Check sheet for the modelled part. Datum: model origin and axes. Units: mm. Face numbers are marked on the shaded views. A direction names the side the tool comes from. Round coordinates to 2 decimals unless told otherwise and drop trailing zeros. Write each loop counter-clockwise with the first axis right and the second up, starting at its lowest first coordinate (ties: lowest second). Pieces come first, ordered by that corner, then holes.
from build123d import *

# Parameters (mm, degrees)
BOSS_EXTRUDE1_DEPTH      = 12.5
BOSS_EXTRUDE1_DEPTH_BACK = 2.5
F_3DSKETCH2_R            = 4.5
CUT_EXTRUDE2_DEPTH       = 1
CUT_EXTRUDE3_REACH       = 68.802
SKETCH3_R                = 3.75
CUT_EXTRUDE6_OUTLINE_R   = 3.25
CUT_EXTRUDE6_DEPTH       = 10
CUT_EXTRUDE7_DEPTH       = 2.5
FILLET1_R                = 5
FILLET2_R                = 4
FILLET3_R                = 4
FILLET4_R                = 3
FILLET5_R                = 3
FILLET6_R                = 4


# Read off the part's stored shape, not the designer's step: Cut-Extrude6
with BuildPart() as part:
    # Sketch1 → Boss-Extrude1 (new, two sides: drawn at the far end of the back side and taken through both)
    with BuildSketch(Plane.XY.offset(-BOSS_EXTRUDE1_DEPTH_BACK)):
        Polygon((0, -8), (0, -32), (-3.5, -32), (-3.5, -64), (0, -64), (0, -38), (7, -38), (7, -20), (12, -20), (12, -8), align=None)
    extrude(amount=BOSS_EXTRUDE1_DEPTH + BOSS_EXTRUDE1_DEPTH_BACK)

    # 3DSketch2 → Cut-Extrude2 (cut)
    with BuildSketch(Plane(origin=(-3.5, -54, 5), x_dir=(0, -1, 0), z_dir=(-1, 0, 0))):
        with Locations(Location((0, 0, 0), (0, 0, 270))):
            Circle(F_3DSKETCH2_R)
    extrude(amount=-CUT_EXTRUDE2_DEPTH, mode=Mode.SUBTRACT)

    # Sketch3 → Cut-Extrude3 (cut, up to next)
    with BuildSketch(Plane.ZY.offset(2.5), mode=Mode.PRIVATE) as cut_extrude3_sk1:
        with Locations((5, -54)):
            Circle(SKETCH3_R)
    cut_extrude3_tool1 = extrude(cut_extrude3_sk1.sketch, amount=-CUT_EXTRUDE3_REACH, mode=Mode.PRIVATE) & part.part
    add(cut_extrude3_tool1.solids().sort_by_distance((-2.5, -54, 5))[0], mode=Mode.SUBTRACT)

    # Cut-Extrude6 outline → Cut-Extrude6 (cut)
    with BuildSketch(Plane.YZ):
        with Locations((-16.5, 5)):
            Circle(CUT_EXTRUDE6_OUTLINE_R)
    extrude(amount=CUT_EXTRUDE6_DEPTH, mode=Mode.SUBTRACT)

    # Sketch4 → Cut-Extrude7 (cut)
    with BuildSketch(Plane.ZY.offset(3.5)):
        with BuildLine():
            Line((5, -46.75), (5, -45.75))
            ThreePointArc((5, -45.75), (4.24685511, -45.784449332), (3.5, -45.88750963))
            Line((3.5, -45.88750963), (3.5, -46.75))
            Line((3.5, -46.75), (5, -46.75))
        make_face()
        with BuildLine():
            ThreePointArc((6.5, -45.88750963), (5.75314489, -45.784449332), (5, -45.75))
            Line((5, -45.75), (5, -46.75))
            Line((5, -46.75), (6.5, -46.75))
            Line((6.5, -46.75), (6.5, -45.88750963))
        make_face()
    extrude(amount=-CUT_EXTRUDE7_DEPTH, mode=Mode.SUBTRACT)

    # Fillet1
    # the kernel refuses this fillet: 5 mm, written as the material it takes off along each edge
    with BuildSketch(Plane(origin=(7, -38, -15), x_dir=(-1, 0, 0), z_dir=(0, 0, 1))) as fillet1_piece_1:
        with BuildLine():
            CenterArc((FILLET1_R, -FILLET1_R), FILLET1_R, 90, 90)
            Line((0, -FILLET1_R), (-FILLET1_R * 0.02, -FILLET1_R))
            Line((-FILLET1_R * 0.02, -FILLET1_R), (-FILLET1_R * 0.02, FILLET1_R * 0.02))
            Line((-FILLET1_R * 0.02, FILLET1_R * 0.02), (FILLET1_R, FILLET1_R * 0.02))
            Line((FILLET1_R, FILLET1_R * 0.02), (FILLET1_R, 0))
        make_face()
    extrude(amount=40, mode=Mode.SUBTRACT)
    with BuildSketch(Plane(origin=(24.5, -8, 12.5), x_dir=(0, 0, -1), z_dir=(-1, 0, 0))) as fillet1_piece_2:
        with BuildLine():
            CenterArc((FILLET1_R, FILLET1_R), FILLET1_R, 180, 90)
            Line((0, FILLET1_R), (-FILLET1_R * 0.02, FILLET1_R))
            Line((-FILLET1_R * 0.02, FILLET1_R), (-FILLET1_R * 0.02, -FILLET1_R * 0.02))
            Line((-FILLET1_R * 0.02, -FILLET1_R * 0.02), (FILLET1_R, -FILLET1_R * 0.02))
            Line((FILLET1_R, -FILLET1_R * 0.02), (FILLET1_R, 0))
        make_face()
    extrude(amount=37, mode=Mode.SUBTRACT)
    with BuildSketch(Plane(origin=(24.5, -8, -2.5), x_dir=(0, 0, 1), z_dir=(-1, 0, 0))) as fillet1_piece_3:
        with BuildLine():
            CenterArc((FILLET1_R, -FILLET1_R), FILLET1_R, 90, 90)
            Line((0, -FILLET1_R), (-FILLET1_R * 0.02, -FILLET1_R))
            Line((-FILLET1_R * 0.02, -FILLET1_R), (-FILLET1_R * 0.02, FILLET1_R * 0.02))
            Line((-FILLET1_R * 0.02, FILLET1_R * 0.02), (FILLET1_R, FILLET1_R * 0.02))
            Line((FILLET1_R, FILLET1_R * 0.02), (FILLET1_R, 0))
        make_face()
    extrude(amount=37, mode=Mode.SUBTRACT)
    with BuildSketch(Plane(origin=(-3.5, -32, -14.424240018), x_dir=(1, 0, 0), z_dir=(0, 0, 1))) as fillet1_piece_4:
        with BuildLine():
            CenterArc((5, -4.769696007), FILLET1_R, 107.457603124, 72.542396876)
            Line((0, -4.769696007), (-0.1, -4.769696007))
            Line((-0.1, -4.769696007), (-0.1, 0))
            Line((-0.1, 0), (0, 0.1))
            ThreePointArc((0, 0.1), (1.75, 0.1), (3.47, 0.09539392))
            Line((3.47, 0.09539392), (3.5, 0))
        make_face()
    extrude(amount=38.848480035, mode=Mode.SUBTRACT)

    # Fillet2
    fillet2_edges = [part.edges().sort_by_distance(p)[0] for p in [
        (0, -32, 5),
    ]]
    fillet(fillet2_edges, radius=FILLET2_R)

    # Fillet3
    fillet3_edges = [part.edges().sort_by_distance(p)[0] for p in [
        (0, -38, 5),
    ]]
    fillet(fillet3_edges, radius=FILLET3_R)

    # Fillet4
    fillet4_edges = [part.edges().sort_by_distance(p)[0] for p in [
        (-1.75, -64, 12.5),
        (-1.75, -64, -2.5),
    ]]
    fillet(fillet4_edges, radius=FILLET4_R)

    # Fillet5
    fillet5_edges = [part.edges().sort_by_distance(p)[0] for p in [
        (12, -20, 5),
    ]]
    fillet(fillet5_edges, radius=FILLET5_R)

    # Fillet6
    fillet6_edges = [part.edges().sort_by_distance(p)[0] for p in [
        (7, -20, 5),
    ]]
    fillet(fillet6_edges, radius=FILLET6_R)


solid = part.part
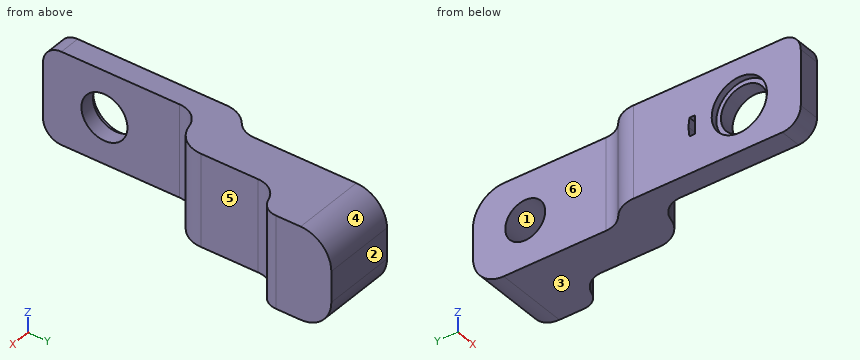
1. Release check for a two-part mould opening along Y. For the marked faces 1, 2 and 3 record: released by +Y, released by -Y, zero draft, split by the parting line, or undercut.
2. Go/stop test with flat-tipped pins: pin 1 (7 mm diameter, centred on y = -54, z = 5, fed in from +X); pin 2 (1.5 mm diameter, centred on x = 3.5, z = 2.5, fed in from -Y); pin 3 (7 mm diameter, centred on y = -17, z = 4, fed in from -X); pin 4 (5 mm diameter, centred on y = -38.5, z = 10.5, fed in from +X). Record where each tip stops, or that it passes through.
3. Scan lines: line 1 along X through (y, z) = (-10.5, 5.5); line 2 along X through (y, z) = (-49.5, 11.5); line 3 along Y through (x, z) = (2.5, 2.75). Record each from-to range of solid material in increasing order.
4. Sectioned sample at A-A, the plane y = -54. Enter the section's corners in (x, z).
5. Sectioned sample at D-D, the plane y = -24.5. Enter the section's corners in (x, z).
6. Set-up check for the marked faces 4, 5 and 6: record each of +Z, -Z, +X, -X, +Y, -Y from which the full face is reachable in a straight line by a thin tool's end or side.
7. Sectioned sample at C-C, the plane y = -16.5. Enter the section's corners in (x, z), plus the area to 3 significant figures.
8. Sectioned sample at B-B, the plane x = 4. Enter the section's corners in (y, z).
Computed values:
1. face 1: undercut
1. face 2: released by +Y
1. face 3: zero draft
2. pin 1: passes through
2. pin 2: stops at y = -37.98
2. pin 3: stops at x = 0
2. pin 4: stops at x = 6
3. line 1: x = 0 to 12
3. line 2: x = -3.5 to 0
3. line 3: y = -38.07 to -18.85, -14.15 to -8
4. outline: (-3.5, -2.5) - (0, -2.5) - (0, 1.25) - (-2.5, 1.25) - (-2.5, 0.5) - (-3.5, 0.5) - close; (-3.5, 9.5) - (-2.5, 9.5) - (-2.5, 8.75) - (0, 8.75) - (0, 12.5) - (-3.5, 12.5) - close
5. outline: (0, -2.5) - (7, -2.5) - (7, 12.5) - (0, 12.5) - close
6. face 4: +Z, +X, -X, +Y
6. face 5: +Z, -Z, +X, -Y
6. face 6: +Z, -Z, -X, +Y
7. outline: (0, -2.5) - (12, -2.5) - (12, 12.5) - (0, 12.5) - (0, 8.25) - (10, 8.25) - (10, 1.75) - (0, 1.75) - close
7. area: 115 mm2
8. outline: (-37.58, -2.5) - (-13, -2.5) arc R5 ccw to (-8, 2.5) - (-8, 7.5) arc R5 ccw to (-13, 12.5) - (-37.58, 12.5) - close; hole circle Ø6.5 at (-16.5, 5)
